Verification items for this drawing (mm, ordinates from the low corner). A direction names the side the tool comes from. Coordinates: 2 decimals unless noted, no trailing zeros. Loops run counter-clockwise (first coordinate to the right, second up) from the corner with the lowest first, then second, coordinate; pieces in that order, holes last. Notation, with made-up numbers: M 16.5,2.25 L 66.5,2.25 A10 ccw 66.5,10.25 Z; hole C 35,-24 d10. An arc over 180 degrees is marked long. Return JSON: item names as keys, results as strings.
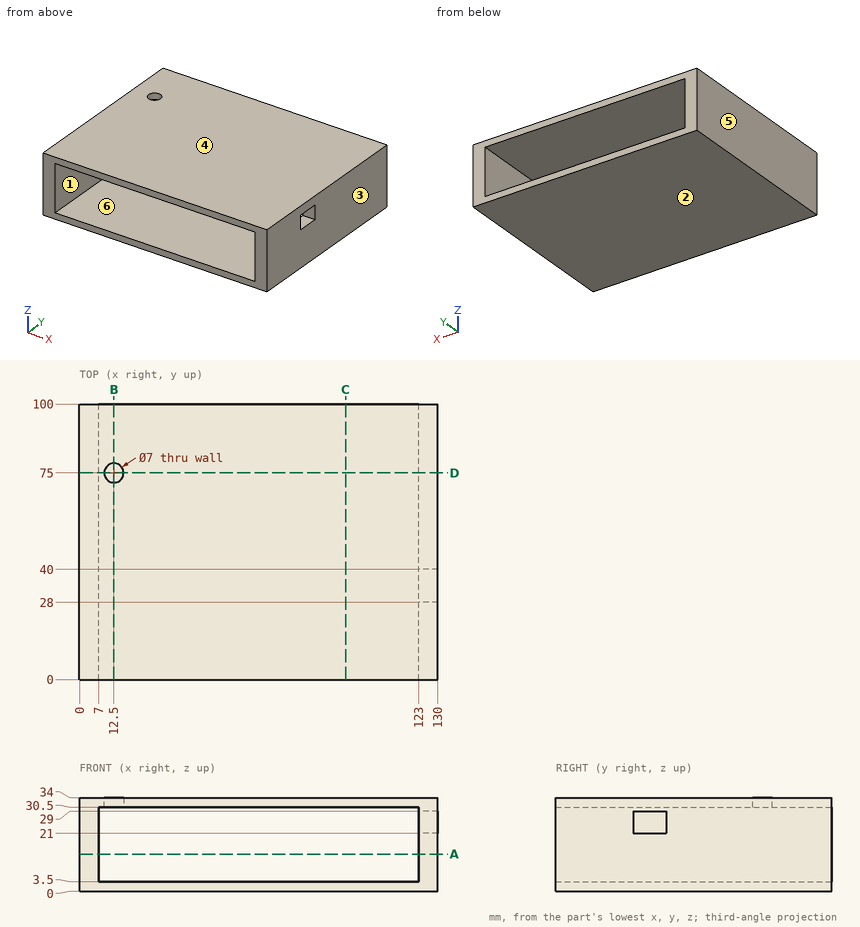
1) Section check C-C on x = 96.5. Record the cut outline in (y, z).
Answers:
{"outline": "M 0,0 L 100,0 L 100,3.5 L 0,3.5 Z; M 0,30.5 L 100,30.5 L 100,34 L 0,34 Z"}
2) Section check B-B on x = 12.5. Record the cut outline in (y, z).
Answers:
{"outline": "M 0,0 L 100,0 L 100,3.5 L 0,3.5 Z; M 0,30.5 L 71.5,30.5 L 71.5,34 L 0,34 Z; M 78.5,30.5 L 100,30.5 L 100,34 L 78.5,34 Z"}
3) Set-up check for the marked faces 5 and 6: record each of +Z, -Z, +X, -X, +Y, -Y from which the full face is reachable in a straight line by a thin tool's end or side.
Answers:
{"face 5": "+Z, -Z, -X, +Y, -Y", "face 6": "+Y, -Y"}
4) Section check A-A on z = 13.5. Record the cut outline in (x, y).
Answers:
{"outline": "M 0,0 L 7,0 L 7,100 L 0,100 Z; M 123,0 L 130,0 L 130,100 L 123,100 Z"}
5) Scan lines: line 1 along Z through (x, y) = (54, 49.5); line 2 along X through (y, z) = (46.5, 11); line 3 along Y through (x, z) = (12.5, 32.6). Record each from-to range of solid material in increasing order. Write a range as [from, to].
Answers:
{"line 1": "[0, 3.5], [30.5, 34]", "line 2": "[0, 7], [123, 130]", "line 3": "[0, 71.5], [78.5, 100]"}
6) Go/stop test with a flat-tipped pin: pin 1 Ø12 at (x, z) = (57, 13) entering from -Y. Record where the tip stops, or that it passes through.
Answers:
{"pin 1": "through"}
7) Section check D-D on y = 75. Record the cut outline in (x, z).
Answers:
{"outline": "M 0,0 L 130,0 L 130,34 L 16,34 L 16,30.5 L 123,30.5 L 123,3.5 L 7,3.5 L 7,30.5 L 9,30.5 L 9,34 L 0,34 Z"}
8) Draft check along Z on the marked faces 1, 2, 3 and 4. Enter one of: +Z half, -Z half, draft (parallel to the pull), parting line (faces both ways), or undercut.
Answers:
{"face 1": "undercut", "face 2": "-Z half", "face 3": "draft", "face 4": "+Z half"}
